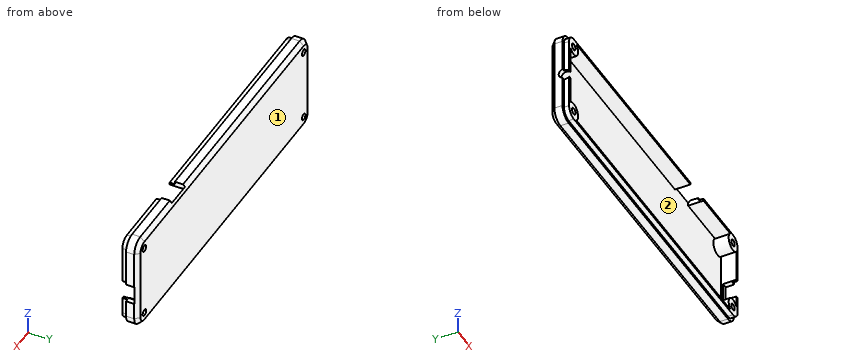
```python
from build123d import *

# Parameters (mm, degrees)
SKETCH037_W       = 7.5
SKETCH037_H       = 7.5
EXTRUDE045_DEPTH  = 10
SKETCH036_W       = 10
SKETCH036_H       = 9
EXTRUDE044_DEPTH  = 10
CYLINDER001_R     = 2
CYLINDER001_DEPTH = 10
SKETCH005_R       = 1.3
EXTRUDE003_DEPTH  = 20
EXTRUDE039_DEPTH  = 4
EXTRUDE042_DEPTH  = 0.8
EXTRUDE002_DEPTH  = 6
EXTRUDE037_DEPTH  = 2


with BuildPart() as extrude045:
    # Sketch037 → Extrude045 (new body)
    with BuildSketch(Plane.YZ.offset(35)):
        with Locations((0, 8)):
            Rectangle(SKETCH037_W, SKETCH037_H)
    extrude(amount=EXTRUDE045_DEPTH)


with BuildPart() as extrude045_1:
    # Extrude045 placement: moved
    add(extrude045.part.moved(Location((-9.5, 0, 0))))


with BuildPart() as extrude044:
    # Sketch036 → Extrude044 (new body)
    with BuildSketch(Plane.XY.offset(40)):
        Rectangle(SKETCH036_W, SKETCH036_H)
    extrude(amount=EXTRUDE044_DEPTH)


with BuildPart() as extrude044_1:
    # Extrude044 placement: moved
    add(extrude044.part.moved(Location((0, 0, -15.5))))


with BuildPart() as common_sub:
    # Cylinder001 → Cylinder001 (new body)
    with BuildSketch(Plane(origin=(-92.5, 0, 12), x_dir=(0, 0, 1), z_dir=(-1, 0, 0))):
        Circle(CYLINDER001_R)
    extrude(amount=CYLINDER001_DEPTH)

    # Fusion033: union Extrude045, Extrude044
    add(extrude045_1.part)
    add(extrude044_1.part)


with BuildPart() as sweep001:
    # Sweep001: sweep along a path in Sketch034
    with BuildLine(Plane.XZ.offset(10)) as sweep001_path:
        Line((32, 11.999174), (32, 26.4))
        ThreePointArc((32, 26.4), (30.652691, 29.652691), (27.4, 31))
        Line((27.4, 31), (-60.9, 31))
    # Sketch035 → Sweep001 (sweep)
    with BuildSketch(Plane.YZ):
        Polygon((5.3, 29.4), (3.7, 31), (3.7, 32), (6, 32), (6, 29.4), align=None)
    sweep(path=sweep001_path.line)


with BuildPart() as fusion030:
    # Sketch005 → Extrude003 (new body)
    with BuildSketch(Plane.XZ.offset(5)):
        with Locations((27.4, 26.4)):
            Circle(SKETCH005_R)
    extrude(amount=-EXTRUDE003_DEPTH)


with BuildPart() as fusion030_1:
    # Extrude003 placement: moved
    add(fusion030.part.moved(Location((0, -4, 0))))

    # Fusion030: union Sweep001
    add(sweep001.part)


with BuildPart() as top003:
    # Sketch028 → Extrude039 (new body)
    with BuildSketch(Plane.XZ.offset(10)):
        with BuildLine():
            ThreePointArc((32, 26.4), (30.652691, 29.652691), (27.4, 31))
            Line((27.4, 31), (-60.9, 31))
            Line((-60.9, 31), (-60.9, 29))
            Line((-60.9, 29), (27.4, 29))
            ThreePointArc((30, 26.4), (29.238478, 28.238478), (27.4, 29))
            Line((30, 12), (30, 26.4))
            Line((32, 12), (30, 12))
            Line((32, 26.4), (32, 12))
        make_face()
    extrude(amount=EXTRUDE039_DEPTH)


with BuildPart() as top003_1:
    # Extrude039 placement: moved
    add(top003.part.moved(Location((0, 14.5, 0))))


with BuildPart() as top002:
    # Sketch031 → Extrude042 (new body)
    with BuildSketch(Plane.XZ.offset(10)):
        with BuildLine():
            ThreePointArc((32, 26.399981), (30.652691, 29.652672), (27.4, 30.999981))
            Line((27.4, 30.999981), (-60.9, 30.999981))
            Line((-60.9, 30.999981), (-60.9, 11.999981))
            Line((-60.9, 11.999981), (32, 11.999981))
            Line((32, 26.399981), (32, 11.999981))
        make_face()
    extrude(amount=EXTRUDE042_DEPTH)


with BuildPart() as top002_1:
    # Extrude042 placement: moved
    add(top002.part.moved(Location((0, 15.3, 0))))


with BuildPart() as screw_hole_top:
    # Sketch004 → Extrude002 (new body)
    with BuildSketch(Plane.XZ.offset(10)):
        with BuildLine():
            ThreePointArc((25.36776, 29), (25.066548, 24.066548), (30, 24.36776))
            Line((30, 24.36776), (30, 26.4))
            ThreePointArc((30, 26.4), (29.238478, 28.238478), (27.4, 29))
            Line((25.36776, 29), (27.4, 29))
        make_face()
    extrude(amount=-EXTRUDE002_DEPTH)


with BuildPart() as screw_hole_top_1:
    # Extrude002 placement: moved
    add(screw_hole_top.part.moved(Location((0, 8.5, 0))))


with BuildPart() as top:
    # Sketch029 → Extrude037 (new body)
    with BuildSketch(Plane.XZ.offset(10)):
        with BuildLine():
            ThreePointArc((30.9, 26.4), (29.874874, 28.874874), (27.4, 29.9))
            Line((27.4, 29.9), (-33, 29.9))
            Line((-33, 29.9), (-33, 29))
            Line((-33, 29), (27.4, 29))
            ThreePointArc((30, 26.4), (29.238478, 28.238478), (27.4, 29))
            Line((30, 12), (30, 26.4))
            Line((30.9, 12), (30, 12))
            Line((30.9, 26.4), (30.9, 12))
        make_face()
    extrude(amount=EXTRUDE037_DEPTH)


with BuildPart() as top_1:
    # Extrude037 placement: moved
    add(top.part.moved(Location((0, 10.5, 0))))

    # Fusion028: union top003, top002, screw hole top
    add(top003_1.part)
    add(top002_1.part)
    add(screw_hole_top_1.part)

    # Cut024: cut Fusion030
    add(fusion030_1.part, mode=Mode.SUBTRACT)


with BuildPart() as part_mirroring:
    # Part__Mirroring: instance of top
    add(top_1.part.mirror(Plane(origin=(0, 0, 12), x_dir=(0, 1, 0), z_dir=(0, 0, 1))))


with BuildPart() as part_mirroring002:
    # Part__Mirroring002: instance of Part__Mirroring
    add(part_mirroring.part.mirror(Plane(origin=(-33, 1, 0), x_dir=(0, -1, 0), z_dir=(1, 0, 0))))


with BuildPart() as top007:
    # Part__Mirroring003: instance of top
    add(top_1.part.mirror(Plane(origin=(-33, 0, 0), x_dir=(0, -1, 0), z_dir=(1, 0, 0))))

    # Fusion032: union top, Part__Mirroring, Part__Mirroring002
    add(top_1.part)
    add(part_mirroring.part)
    add(part_mirroring002.part)

    # Cut025: cut common sub
    add(common_sub.part, mode=Mode.SUBTRACT)


solid = top007.part
```
Source: CAD feature listing. Evaluate the final solid. Frame: model axes, mm. Face numbers are marked on the shaded views. Coordinates: 2 decimals unless noted, no trailing zeros. Write each loop counter-clockwise with the first axis right and the second up, starting at its lowest first coordinate (ties: lowest second). Pieces come first, ordered by that corner, then holes. Notation, with made-up numbers: (15.25, 79.5) -> (33.25, 79.5) arc R21 ccw to (33.25, 108.5) -> close; hole circle Ø6 at (-4.5, 38). An arc over 180 degrees is marked (long way). Return JSON: item names as keys, results as strings. Group by question number.
1) Ray query, line 1 along Z through (x, y) = (27.4, 2.5); line 2 along Z through (x, y) = (-27, 1); line 3 along Y through (x, z) = (-59, 12). Return the intervals inside material, ascending.
2) Contact query for flat-ended pins moving along their axis: P1, Ø6, axis at x = 10.5, z = 22.5, coming from the -Y side; P2, Ø2, axis at y = -1, z = 2, coming from the +X side; P3, Ø0.6, axis at x = -17, y = -1, coming from the -Z side. Output: stop coordinate, or through.
3) Section query A-A, the plane x = -32.5. Return loops of the section in (y, z), plus the area to 3 significant figures.
4) Mould query, pull axis Z, two halves, no side actions, for the marked faces 1 and 2. Classes: +Z half, -Z half, draft (parallel to the pull), parting line (faces both ways), or undercut.
From the geometry:
{
 "1": {"line 1": "-7 to -3.7, -1.1 to 0.9, 23.1 to 25.1, 27.7 to 31", "line 2": "-7 to -5, 29 to 31", "line 3": "4.5 to 5.3"},
 "2": {"P1": "y = 4.5", "P2": "x = 30.9", "P3": "z = -5.9"},
 "3": {"outline": "(-1.5, -5.9) -> (0.5, -5.9) -> (0.5, -7) -> (3.7, -7) -> (5.3, -5.4) -> (5.3, 29.4) -> (3.7, 31) -> (0.5, 31) -> (0.5, 29.9) -> (-1.5, 29.9) -> (-1.5, 29) -> (4.5, 29) -> (4.5, -5) -> (-1.5, -5) -> close", "area": "47.4 mm²"},
 "4": {"face 1": "draft", "face 2": "undercut"}
}
